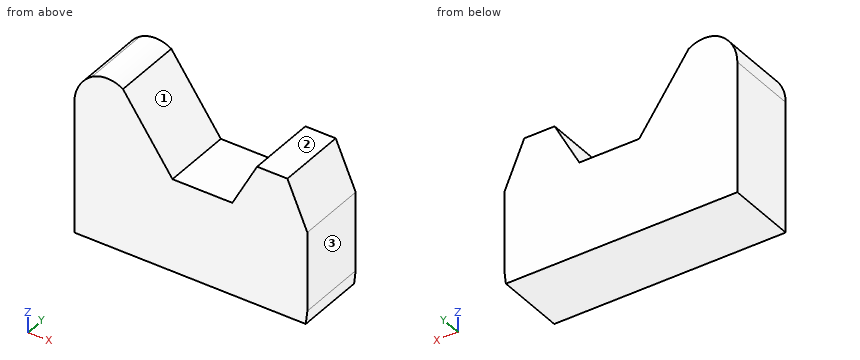
```python
from build123d import *

# Parameters (mm, degrees)
F1_DEPTH = 19.304


# Not quite as in the source:
# - the program builds the solid bodies; features that only make, move or delete a surface that nothing else refers to are left out


with BuildPart() as f1:
    # F0 (on Front) → F1 (new body)
    with BuildSketch(Plane.XZ):
        with BuildLine():
            Line((-26.9875, 34.112624824), (-26.9875, 1.898483652))
            Line((-26.9875, 1.898483652), (26.9875, 1.898483652))
            Line((26.9875, 1.898483652), (37.0624177158, 1.8666714896))
            Line((37.0624177158, 1.8666714896), (37.0624177158, 23.583335802))
            Line((37.0624177158, 23.583335802), (31.5784178674, 36.2954275192))
            Line((31.5784178674, 36.2954275192), (23.2427231967, 36.2954275192))
            Line((23.2427231967, 36.2954275192), (16.4425540715, 23.583335802))
            Line((16.4425540715, 23.583335802), (0, 23.583335802))
            Line((0, 23.583335802), (-13.6097995564, 43.0830909645))
            ThreePointArc((-13.6097995564, 43.0830909645), (-17.8935738167, 44.3218275192), (-22.177348077, 43.0830909645))
            ThreePointArc((-22.177348077, 43.0830909645), (-25.7090842299, 39.2019966984), (-26.9875, 34.112624824))
        make_face()
        Polygon((26.9875, 1.898483652), (-26.9875, 1.898483652), (-26.9875, -1.898483652), (26.9875, -1.898483652), (36.6236940026, -1.898483652), (37.0624177158, 1.8666714896), align=None)
    extrude(amount=F1_DEPTH)


solid = f1.part
```
Could you check a few things on this model? Use its own coordinates, in mm. Face numbers are marked on the shaded views. A direction names the side the tool comes from. Round coordinates to 2 decimals unless told otherwise and drop trailing zeros. Write each loop counter-clockwise with the first axis right and the second up, starting at its lowest first coordinate (ties: lowest second). Pieces come first, ordered by that corner, then holes. Notation, with made-up numbers: M -16,-6.5 L 1,-6.5 A17 cw 1,17.5 Z; hole C 0,-7.75 d5. An arc over 180 degrees is marked long. Answer in a Markdown table with one row per item. Add a question column.
Q1. Imagine slicing it at B-B (z = 26). Please give me the cut outline in (x, y), then the cut area to 3 significant figures.
Q2. Imagine slicing it at A-A (y = -13.75). Please give me the cut outline in (x, z).
Q3. If I drill on line 1 (Z direction, x = 30.5, y = -8.5); line 2 (X direction, y = -3.75, z = 27); line 3 (Z direction, x = 2, y = -6.75), over which ranges is the centre line in solid material (lowest first)? Write a range as from..to.
Q4. Imagine slicing it at C-C (x = 3.5). Please give me the cut outline in (y, z), then the cut area to 3 significant figures.
Q5. Imagine slicing it at D-D (z = 39). Please give me the cut outline in (x, y).
Q6. On a 3-axis mill with a long thin cutter (end or side, diameter ignored), from which of +Z, -Z, +X, -X, +Y, -Y can I reach the whole of each face in a straight line? I mean the marked faces 1, 2 and 3. Say none if no direction works.
Q7. Will this pin go through, and if not, where does the flat tip stop? pin 1 Ø3 at (x, y) = (30, -17.5) entering from +Z.
Values:
| question | item | result |
|---|---|---|
| 1 | outline | M -26.99,-19.3 L -1.69,-19.3 L -1.69,0 L -26.99,0 Z; M 17.74,-19.3 L 36.02,-19.3 L 36.02,0 L 17.74,0 Z |
| 1 | area | 841 mm^2 |
| 2 | outline | M -26.99,-1.9 L 36.62,-1.9 L 37.06,1.87 L 37.06,23.58 L 31.58,36.3 L 23.24,36.3 L 16.44,23.58 L 0,23.58 L -13.61,43.08 A8.03 ccw -22.18,43.08 A10.77 ccw -26.99,34.11 Z |
| 3 | line 1 | -1.9..36.3 |
| 3 | line 2 | -26.99..-2.38, 18.27..35.59 |
| 3 | line 3 | -1.9..23.58 |
| 4 | outline | M -19.3,-1.9 L 0,-1.9 L 0,23.58 L -19.3,23.58 Z |
| 4 | area | 492 mm^2 |
| 5 | outline | M -25.81,-19.3 L -10.76,-19.3 L -10.76,0 L -25.81,0 Z |
| 6 | face 1 | +Z, +Y, -Y |
| 6 | face 2 | +Z, +X, +Y, -Y |
| 6 | face 3 | +Z, -Z, +X, +Y, -Y |
| 7 | pin 1 | z = 36.3 |
